For this review, take the finished solid that the model builds, in its own axes (mm). Face numbers are marked on the shaded views. A direction names the side the tool comes from. Give positions to 0.01 mm unless a question says otherwise; leave off trailing zeros. Write each loop counter-clockwise with the first axis right and the second up, starting at its lowest first coordinate (ties: lowest second). Pieces come first, ordered by that corner, then holes.
Q1. For line 1 (Z direction, x = -2.25, y = 0); line 2 (X direction, y = 1.75, z = -43); line 3 (Y direction, x = -1.05, z = 0), list the stretches that pass through material, from the lowest coordinate up.
Q2. We need section C-C (z = -43). Write out the cut boundary in (x, y), then the cut area to 3 significant figures.
Q3. Machinability: for the marked faces 5, 6 and 7, which of the approach directions +Z, -Z, +X, -X, +Y, -Y give a long, thin tool a straight path to every point of the face, cutting with its end or side? Answer none if there is none.
Q4. We need section B-B (y = 0). Write out the cut boundary in (x, z).
Q5. We need section A-A (x = -5.25). Write out the cut boundary in (y, z).
Q6. Mouldability with a two-part tool opening along X and no side actions: class the marked faces 1, 2, 3 and 4 as released by +X, released by -X, zero draft, split by the parting line, or undercut.
Q7. Insertion check: P1, Ø2, axis at x = 5.5, y = 1.5, coming from the +Z side; P2, Ø3, axis at y = 0.5, z = -24.5, coming from the -X side; P3, Ø4.5, axis at y = 0.5, z = -10.5, coming from the +X side. Each pin has a flat end and moves straight along its axis. Give the tip position at first contact, or say it passes through.
Q8. We need section D-D (z = -19). Write out the cut boundary in (x, y), then the cut area to 3 significant figures.
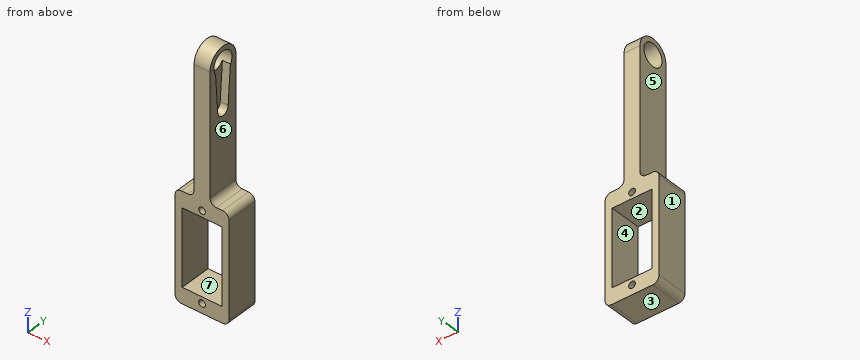
Autodesk Inventor part; units mm, degrees
ref_plane "YZ Plane" through (0, 0, 0) normal (1, 0, 0) x (0, 1, 0)
ref_plane "XZ Plane" through (0, 0, 0) normal (0, 1, 0) x (-1, 0, 0)
ref_plane "XY Plane" through (0, 0, 0) normal (0, 0, 1) x (1, 0, 0)
sketch "Sketch2" plane through (0, 0, 0) normal (1, 0, 0) x (0, 1, 0)
  circle A0 centre (0, 0) radius 3.5
  line L0 (5, 0) -> (5, -40)
  line L1 (5, -40) -> (-5, -40)
  line L2 (-5, -40) -> (-5, 0)
  line L3 (-5, 0) -> (5, 0) construction
  arc A1 (5, 0) -> (-5, 0) centre (0, 0) ccw
  line L4 (0, 0) -> (5, 0) construction
  line L5 (0, 0) -> (0, 5) construction
  line L6 (0, 0) -> (-5, 0) construction
  point P0 (-5, 0)
  dimension "d1" = 7
  dimension "d2" = 5
  dimension "d3" = 90
  dimension "d4" = 180
  dimension "d11" = 40
extrude "Extrusion1" add sketch "Sketch2" along normal mid plane 5
sketch "Sketch4" plane through (-2.5, 5, 0) normal (0, 1, 0) x (1, 0, 0)
  line L0 (2.5, 89.8) -> (2.5, -20.8)
  line L1 (-9.4, 0) -> (14.4, 0)
  line L2 (-6, 74) -> (11, 74)
  line L3 (11, 74) -> (11, 40)
  line L4 (11, 40) -> (-6, 40)
  line L5 (-6, 40) -> (-6, 74)
  line L6 (-6, 57) -> (11, 57) construction
  line L7 (-3.75, 69) -> (8.75, 69)
  line L8 (8.75, 69) -> (8.75, 45)
  line L9 (8.75, 45) -> (-3.75, 45)
  line L10 (-3.75, 45) -> (-3.75, 69)
  line L11 (-3.75, 69) -> (8.75, 45) construction
  line L12 (8.75, 69) -> (-3.75, 45) construction
  line L13 (5, 40) -> (0, 40)
  line L14 (2.5, 71) -> (2.5, 43) construction
  circle A0 centre (2.5, 71) radius 1.05
  circle A1 centre (2.5, 43) radius 1.05
  point P0 (2.5, 0)
  point P1 (2.5, 57)
  point P2 (2.5, 40)
  point P3 (2.5, 57)
  dimension "d18" = 34
  dimension "d19" = 17
  dimension "d20" = 12.5
  dimension "d21" = 24
  dimension "d22" = 2.1
  dimension "d23" = 28
extrude "Extrusion3" add sketch "Sketch4" against normal up to surface (10 mm away) contours L2 L3 L4 L0 A1 L9 L8 L7 A0 | L0 A0 L7 L10 L9 A1 L4 L5 L2
sketch "Sketch5" plane through (2.5, 0, 0) normal (1, 0, 0) x (0, 0, -1)
  circle A0 centre (0, 0) radius 3
  arc A1 (14, -2) -> (14, 2) centre (14, 0) ccw
  line L0 (14, 0) -> (14, 2) construction
  line L1 (14, 0) -> (16, 0) construction
  line L2 (14, 0) -> (14, -2) construction
  line L3 (0, 11.9) -> (0, -11.9)
  line L4 (14, 2) -> (0, 3)
  line L5 (14, -2) -> (0, -3)
  point P0 (0.4264, -2.9695)
  point P1 (0.4264, 2.9695)
  dimension "d27" = 6
  dimension "d28" = 90
  dimension "d29" = 180
  dimension "d30" = 14
  dimension "d31" = 2
fillet "Fillet1" radius 2 6 edges at (2.5, 0, -40) (8.5, 0, -40) (8.5, 0, -74) (-8.5, 0, -74) (-8.5, 0, -40) (-2.5, 0, -40)
extrude "Extrusion4" cut sketch "Sketch5" against normal blind 2.5
properties part number "link3"
Computed:
1. line 1: z = -74 to -69, -45 to -3.5, 3.5 to 5
1. line 2: x = -8.5 to -1.05, 1.05 to 8.5
1. line 3: y = -5 to -3.5, 3.5 to 5
2. outline: (-8.5, -5) - (-1.05, -5) - (-1.05, 5) - (-8.5, 5) - close; (1.05, -5) - (8.5, -5) - (8.5, 5) - (1.05, 5) - close
2. area: 149 mm2
3. face 5: +Z, -X, +Y, -Y
3. face 6: +Z, +X, +Y, -Y
3. face 7: +Y, -Y
4. outline: (-8.5, -72) arc R2 ccw to (-6.5, -74) - (6.5, -74) arc R2 ccw to (8.5, -72) - (8.5, -42) arc R2 ccw to (6.5, -40) - (4.5, -40) arc R2 cw to (2.5, -38) - (2.5, -16) - (0, -16) - (0, -3.5) - (-2.5, -3.5) - (-2.5, -38) arc R2 cw to (-4.5, -40) - (-6.5, -40) arc R2 ccw to (-8.5, -42) - close; (-2.5, 3.5) - (2.5, 3.5) - (2.5, 5) - (-2.5, 5) - close; hole (-6.25, -69) - (6.25, -69) - (6.25, -45) - (-6.25, -45) - close; hole circle Ø2.1 at (0, -71); hole circle Ø2.1 at (0, -43)
5. outline: (-5, -74) - (5, -74) - (5, -69) - (-5, -69) - close; (-5, -45) - (5, -45) - (5, -40) - (-5, -40) - close
6. face 1: released by -X
6. face 2: undercut
6. face 3: zero draft
6. face 4: undercut
7. P1: stops at z = -40
7. P2: stops at x = -2.5
7. P3: stops at x = 2.5
8. outline: (-2.5, -5) - (2.5, -5) - (2.5, 5) - (-2.5, 5) - close
8. area: 50.0 mm2
